Could you check a few things on this model? Use its own coordinates, in mm. Face numbers are marked on the shaded views. Give positions to 0.01 mm unless a question says otherwise; leave off trailing zeros. Write each loop counter-clockwise with the first axis right and the second up, starting at its lowest first coordinate (ties: lowest second). Pieces come first, ordered by that corner, then holes. Notation, with made-up numbers: (73, 74) - (91, 74) arc R32 ccw to (91, 112) - close; hole circle Ø1 at (75.5, -19). An arc over 180 degrees is marked (long way). Use one line per item in the form item = value.
```python
from build123d import *

# Parameters (mm, degrees)
PATH_R = 7


with BuildPart() as part:
    # Cam Handle: sweep along a path in Circle
    with BuildLine(Plane.XY) as cam_handle_path:
        Line((0, 0), (5.789702512, 66.176602527))
        ThreePointArc((5.789702512, 66.176602527), (10.117863133, 74.953244047), (19.238330936, 78.5))
        Line((19.238330936, 78.5), (103.782702537, 78.5))
        ThreePointArc((103.782702537, 78.5), (112.90317034, 74.953244047), (117.231330962, 66.176602527))
        Line((117.231330962, 66.176602527), (121.35, 19.1))
    # Path → Cam Handle (sweep)
    with BuildSketch(Plane(origin=(0, 0, 0), x_dir=(0.9961946980917455, -0.08715574274765839, 0), z_dir=(0.0871557427476584, 0.9961946980917457, 0))):
        Circle(PATH_R)
    sweep(path=cam_handle_path.line)


solid = part.part
```
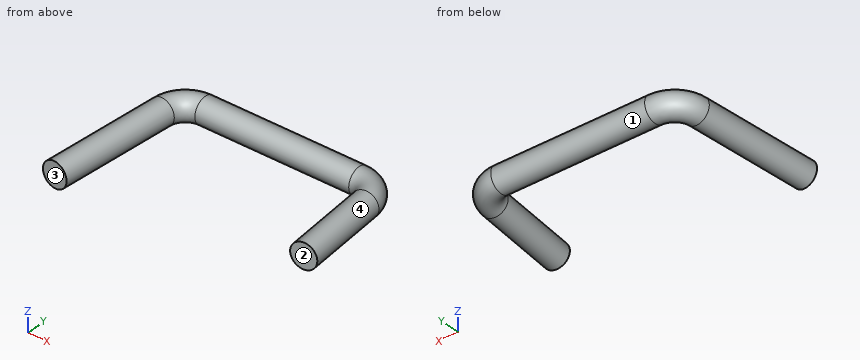
1. For pin 1 (1.5 mm diameter, centred on y = 31.5, z = 4, fed in from +X); pin 2 (8 mm diameter, centred on x = 14, z = -3, fed in from +Y); pin 3 (5 mm diameter, centred on y = 49, z = 5, fed in from +X), each with a flat end and sliding along its axis, tell me the tip position at first contact or that it passes through.
Response values:
pin_1 = 126.49
pin_2 = 85.37
pin_3 = 125.32
2. Imagine slicing it at B-B, the plane x = 69.5. List the corners of the cut face in (y, z) for me.
Response values:
outline = circle Ø14 at (78.5, 0)
3. If I drill on line 1 (Y direction, x = 80.5, z = -0.25); line 2 (X direction, y = 59.5, z = 2.5); line 3 (X direction, y = 20, z = -2.5), over which ranges is the centre line in solid material (lowest first)? Write a range as from..to.
Response values:
line_1 = 71.5..85.5
line_2 = -1.36..11.77, 111.25..124.38
line_3 = -4.81..8.31, 114.71..127.83
4. If we mould it in two halves opening along X, with no side actions, what happens to the marked faces 1, 2, 3 and 4? For each: pulls with the +X half, pulls with the -X half, needs draft (parallel to the pull), parting line crosses it, or undercut.
Response values:
face_1 = undercut
face_2 = pulls with the +X half
face_3 = pulls with the -X half
face_4 = undercut
5. Imagine slicing it at A-A, the plane z = 0. List the corners of the cut face in (x, y) for me, and give its area (3 significant figures).
Response values:
outline = (-6.97, 0.61) - (6.97, -0.61) - (12.76, 65.57) arc R6.5 cw to (19.24, 71.5) - (103.78, 71.5) arc R6.5 cw to (110.26, 65.57) - (114.38, 18.49) - (128.32, 19.71) - (124.2, 66.79) arc R20.5 ccw to (103.78, 85.5) - (19.24, 85.5) arc R20.5 ccw to (-1.18, 66.79) - close
area = 3,340 mm²
